from build123d import *

# Parameters (mm, degrees)
SKETCH1_R           = 1.6
SKETCH1_R_2         = 2.5
BOSS_EXTRUDE1_DEPTH = 1.57
FILLET1_R           = 5
SKETCH2_R           = 2.5
SKETCH2_R_2         = 1.6
BOSS_EXTRUDE2_DEPTH = 2.83
SKETCH3_R           = 5
SKETCH3_R_2         = 1.6
BOSS_EXTRUDE3_DEPTH = 0.6
CUT_EXTRUDE1_START  = -10
CUT_EXTRUDE1_DEPTH  = 10


with BuildPart() as part:
    # Sketch1 → Boss-Extrude1 (new body)
    with BuildSketch(Plane(origin=(0, 0, 0), x_dir=(1, 0, 0), z_dir=(0, 1, 0))):
        Polygon((-5, -5), (30.925365976, -5), (-5, 23.304833799), align=None)
        with Locations(Location((16.5, 0, 0), (0, 0, 270))):
            Circle(SKETCH1_R, mode=Mode.SUBTRACT)
        with Locations(Location((0, 0, 0), (0, 0, 270))):
            Circle(SKETCH1_R_2, mode=Mode.SUBTRACT)
        with Locations(Location((0, 13, 0), (0, 0, 270))):
            Circle(SKETCH1_R, mode=Mode.SUBTRACT)
    extrude(amount=BOSS_EXTRUDE1_DEPTH)

    # Fillet1
    fillet1_edges = [part.edges().sort_by_distance(p)[0] for p in [
        (-5, 0.785, -23.304833799),
        (30.925365976, 0.785, 5),
        (-5, 0.785, 5),
    ]]
    fillet(fillet1_edges, radius=FILLET1_R)

    # Sketch2 → Boss-Extrude2 (add)
    with BuildSketch(Plane(origin=(0, 1.57, 0), x_dir=(1, 0, 0), z_dir=(0, 1, 0))):
        with BuildLine():
            Line((19.594361133, 3.927458361), (3.094361133, 16.927458361))
            ThreePointArc((3.094361133, 16.927458361), (-2.182681188, 17.498433375), (-5, 13))
            Line((-5, 13), (-5, 0))
            ThreePointArc((-5, 0), (-3.535533906, -3.535533906), (0, -5))
            Line((0, -5), (16.5, -5))
            ThreePointArc((16.5, -5), (21.224261413, -1.637484075), (19.594361133, 3.927458361))
        make_face()
        with Locations(Location((0, 0, 0), (0, 0, 270))):
            Circle(SKETCH2_R, mode=Mode.SUBTRACT)
        with Locations(Location((16.5, 0, 0), (0, 0, 270))):
            Circle(SKETCH2_R_2, mode=Mode.SUBTRACT)
        with Locations(Location((0, 13, 0), (0, 0, 270))):
            Circle(SKETCH2_R_2, mode=Mode.SUBTRACT)
    extrude(amount=BOSS_EXTRUDE2_DEPTH)

    # Sketch3 → Boss-Extrude3 (add)
    # profile 1 of 2: a face of its own
    with BuildSketch(Plane.XZ):
        with Locations(Location((16.5, 0, 0), (0, 0, 270))):
            Circle(SKETCH3_R)
        with Locations(Location((16.5, 0, 0), (0, 0, 270))):
            Circle(SKETCH3_R_2, mode=Mode.SUBTRACT)
    # profile 2 of 2: a face of its own
    with BuildSketch(Plane.XZ):
        with Locations(Location((0, -13, 0), (0, 0, 270))):
            Circle(SKETCH3_R)
        with Locations(Location((0, -13, 0), (0, 0, 270))):
            Circle(SKETCH3_R_2, mode=Mode.SUBTRACT)
    extrude(amount=BOSS_EXTRUDE3_DEPTH)

    # Sketch4 → Cut-Extrude1 (cut)
    with BuildSketch(Plane(origin=(0, 4.4, 0), x_dir=(1, 0, 0), z_dir=(0, 1, 0)).offset(CUT_EXTRUDE1_START)):
        with BuildLine():
            Line((2.119130133, -3.026431476), (2.176569541, -3.108463452))
            ThreePointArc((2.176569541, -3.108463452), (2.208718169, -3.263081334), (2.118672771, -3.392819725))
            ThreePointArc((2.118672771, -3.392819725), (-2.828427125, -2.828427125), (-3.392819725, 2.118672771))
            ThreePointArc((-3.392819725, 2.118672771), (-3.263081334, 2.208718169), (-3.108463452, 2.176569541))
            Line((-3.108463452, 2.176569541), (-3.026431476, 2.119130133))
            ThreePointArc((-3.026431476, 2.119130133), (-2.945196197, 1.995341896), (-2.971355046, 1.849607847))
            ThreePointArc((-2.971355046, 1.849607847), (-3.498720526, -0.094629188), (-2.867032155, -2.007517527))
            ThreePointArc((-2.867032155, -2.007517527), (-2.170667915, -2.130305331), (-2.047880111, -1.433941091))
            ThreePointArc((-2.047880111, -1.433941091), (-1.767766953, -1.767766953), (-1.433941091, -2.047880111))
            ThreePointArc((-1.433941091, -2.047880111), (-2.130305331, -2.170667915), (-2.007517527, -2.867032155))
            ThreePointArc((-2.007517527, -2.867032155), (-0.094629188, -3.498720526), (1.849607847, -2.971355046))
            ThreePointArc((1.849607847, -2.971355046), (1.995341896, -2.945196197), (2.119130133, -3.026431476))
        make_face()
    extrude(amount=CUT_EXTRUDE1_DEPTH, mode=Mode.SUBTRACT)


with BuildPart() as body_2:
    # Mirror1: mirrored copy
    add(part.part.mirror(Plane(origin=(-5, 1.57, -23.304833799), x_dir=(0, 0, 1), z_dir=(1, 0, 0))))


solid = body_2.part
Verification items for the finished model (mm, model axes). A direction names the side the tool comes from. Coordinates: 2 decimals unless noted, no trailing zeros. Order: outer loops, then holes, each group sorted by start corner. A loop starts at its lowest first (then second) coordinate and runs counter-clockwise, first axis right, second up. Notation, with made-up numbers: M 52,43.5 L 83,43.5 A13 ccw 83,67.5 Z; hole C -4.5,-7.75 d6. An arc over 180 degrees is marked long. Return JSON: item names as keys, results as strings.
1) Thickness scan on L1, parallel to Z at x = -10, y = 2.85; L2, parallel to X at y = 2.8, z = 0; L3, parallel to X at y = 0.6, z = -1.75. Record the ranges inside material, lowest first. Write a range as [from, to].
Answer list:
{"L1": "[-18, -14.6], [-11.4, -2.5], [2.5, 3.5], [4, 5]", "L2": "[-31.5, -28.1], [-24.9, -12.5], [-7.5, -6.5], [-6, -5]", "L3": "[-31.18, -11.79], [-8.21, -6.97], [-6.4, -5]"}
2) Access from +Z, -Z, +X, -X, +Y, -Y to the whole of each face (thin tool, end or side, straight path). Record for faces 4 (the cylindrical face through (-6.5, 2.2, 0.1)), 5 (the flat face through (-5, 2, -7)).
Answer list:
{"face 4": "+Y, -Y", "face 5": "+Z, -Z, +X, +Y, -Y"}
3) Cross-section at D-D, the plane x = -24.5. Record the boundary of the cut face in (y, z).
Answer list:
{"outline": "M -0.6,-4.58 L 0,-4.58 L 0,-7.94 L 4.4,-7.94 L 4.4,5 L 0,5 L 0,4.58 L -0.6,4.58 Z"}
4) Cross-section at B-B, the plane z = -12. Record the boundary of the cut face in (x, y), and give its area (3 significant figures).
Answer list:
{"outline": "M -19.35,0 L -14.9,0 L -14.9,-0.6 L -11.25,-0.6 L -11.25,4.4 L -19.35,4.4 Z; M -8.75,-0.6 L -5.1,-0.6 L -5.1,0 L -5,0 L -5,4.4 L -8.75,4.4 Z", "area": "56.5 mm2"}
5) Cross-section at C-C, the plane y = 1.2. Record the boundary of the cut face in (x, z), and give its area (3 significant figures).
Answer list:
{"outline": "M -29.59,-3.93 L -13.09,-16.93 A5 ccw -5,-13 L -5,0 A5 ccw -10,5 L -26.5,5 A5 ccw Z; hole C -26.5,0 d3.2; hole M -12.18,3.11 L -12.12,3.03 A0.2 ccw -11.85,2.97 A3.5 cw -7.99,2.87 A0.5 cw -8.57,2.05 A2.5 ccw long -7.95,1.43 A0.5 cw -7.13,2.01 A3.5 cw -7.03,-1.85 A0.2 ccw -6.97,-2.12 L -6.89,-2.18 A0.2 ccw -6.61,-2.12 A4 ccw -12.12,3.39 A0.2 ccw Z; hole C -10,-13 d3.2", "area": "397 mm2"}
6) Gauge pin test, flat ends, axial feed: pin 1 (2 mm diameter, centred on y = 3, z = -10, fed in from -X); pin 2 (1 mm diameter, centred on y = 2, z = -11, fed in from -X); pin 3 (11 mm diameter, centred on x = -19.5, z = -6.5, fed in from -Y); pin 4 (3 mm diameter, centred on x = -19, y = 1, fed in from -Z). Record the tip position at first contact, or that the pin passes through.
Answer list:
{"pin 1": "x = -23.16", "pin 2": "x = -21.25", "pin 3": "y = -0.6", "pin 4": "z = -13.46"}
7) Release check for a two-part mould opening along Z. For faces 1 (the flat face through (-18, 2, 5)), 2 (the cylindrical face through (-11.84, 2.17, -1.69)), 3 (the flat face through (-17, 0, -4)) record: +Z half, -Z half, draft (parallel to the pull), parting line (faces both ways), or undercut.
Answer list:
{"face 1": "+Z half", "face 2": "undercut", "face 3": "draft"}
